Build history of the part. All positions in model axes, mm. Face numbers are marked on the shaded views. A direction names the side the tool comes from. Round coordinates to 2 decimals unless told otherwise and drop trailing zeros. Order: outer loops, then holes, each group sorted by start corner. A loop starts at its lowest first (then second) coordinate and runs counter-clockwise, first axis right, second up. Notation, with made-up numbers: (51.5, -14) - (64.5, -14) arc R14 cw to (64.5, -2) - close; hole circle Ø4 at (-4, -19). An arc over 180 degrees is marked (long way). One line per question, with ' | ' between items. Start each with the question number.
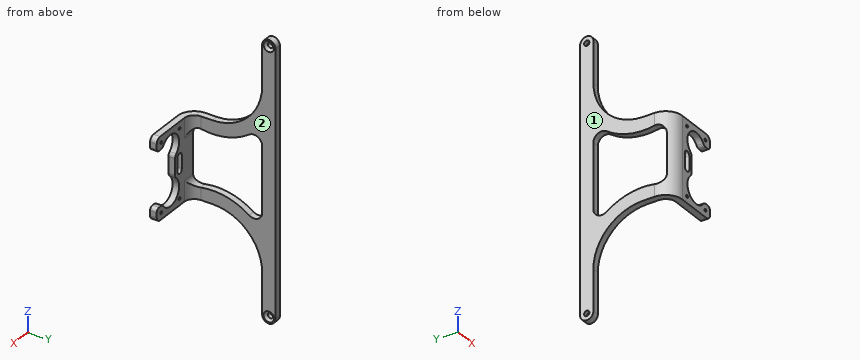
from build123d import *

# Parameters (mm, degrees)
BOSS_EXTRU_1_DEPTH                             = 166
FRAISAGE_POUR_VIS_T_TE_FRAIS_E_M31_D           = 3.2
FRAISAGE_POUR_VIS_T_TE_FRAIS_E_M31_DEPTH       = 4
FRAISAGE_POUR_VIS_T_TE_FRAIS_E_M31_CSINK_D     = 6.3
FRAISAGE_POUR_VIS_T_TE_FRAIS_E_M31_CSINK_ANGLE = 90
D_GAGEMENT_M1_61_D                             = 1.7
D_GAGEMENT_M1_61_DEPTH                         = 4
ENL_V_MAT_EXTRU_1_DEPTH                        = 4
ENL_V_MAT_EXTRU_2_DEPTH                        = 31.75
ENL_V_MAT_EXTRU_2_DEPTH_BACK                   = 5


with BuildPart() as part:
    # Esquisse1 → Boss.-Extru.1 (new body)
    with BuildSketch(Plane.XY):
        with BuildLine():
            Line((0, 0), (-25, 0))
            ThreePointArc((-25, 0), (-32.071067812, 2.928932188), (-35, 10))
            Line((-35, 10), (-35, 55))
            Line((-35, 55), (-31, 55))
            Line((-31, 55), (-31, 10))
            ThreePointArc((-31, 10), (-29.242640687, 5.757359313), (-25, 4))
            Line((-25, 4), (0, 4))
            Line((0, 4), (0, 0))
        make_face()
    extrude(amount=BOSS_EXTRU_1_DEPTH)

    # Fraisage pour vis à tête fraisée M31
    with Locations(Plane(origin=(-31, 0, 0), x_dir=(0, 0, 1), z_dir=(1, 0, 0))):
        with Locations((4, -51), (162, -51)):
            CounterSinkHole(FRAISAGE_POUR_VIS_T_TE_FRAIS_E_M31_D / 2, FRAISAGE_POUR_VIS_T_TE_FRAIS_E_M31_CSINK_D / 2, depth=FRAISAGE_POUR_VIS_T_TE_FRAIS_E_M31_DEPTH, counter_sink_angle=FRAISAGE_POUR_VIS_T_TE_FRAIS_E_M31_CSINK_ANGLE)

    # Dégagement M1.61
    with Locations(Plane(origin=(0, 0, 0), x_dir=(-1, 0, 0), z_dir=(0, -1, 0))):
        with Locations((20.75, -62.5), (20.75, -103.5), (4.25, -103.5), (4.25, -62.5)):
            Hole(D_GAGEMENT_M1_61_D / 2, depth=D_GAGEMENT_M1_61_DEPTH)

    # Esquisse6 → Enlèv. mat.-Extru.1 (cut)
    with BuildSketch(Plane.XZ):
        with BuildLine():
            Line((-35, 58.5), (-3.25, 58.5))
            ThreePointArc((-3.25, 58.5), (-1.128679656, 59.378679656), (-0.25, 61.5))
            Line((-0.25, 61.5), (-0.25, 64.5))
            ThreePointArc((-0.25, 64.5), (-0.835786438, 65.914213562), (-2.25, 66.5))
            Line((-2.25, 66.5), (-3.750142858, 66.5))
            ThreePointArc((-3.750142858, 66.5), (-5.097923909, 66.180202649), (-6.15836042, 65.288990826))
            ThreePointArc((-6.15836042, 65.288990826), (-17.832822404, 64.171534919), (-17.754587156, 75.899094322))
            ThreePointArc((-17.754587156, 75.899094322), (-17.012643745, 76.911706018), (-16.75, 78.139256723))
            Line((-16.75, 78.139256723), (-16.75, 87.860743277))
            ThreePointArc((-16.75, 87.860743277), (-17.012643745, 89.088293982), (-17.754587156, 90.100905678))
            ThreePointArc((-17.754587156, 90.100905678), (-17.832822404, 101.828465081), (-6.15836042, 100.711009174))
            ThreePointArc((-6.15836042, 100.711009174), (-5.097923909, 99.819797351), (-3.750142858, 99.5))
            Line((-3.750142858, 99.5), (-2.25, 99.5))
            ThreePointArc((-2.25, 99.5), (-0.835786438, 100.085786438), (-0.25, 101.5))
            Line((-0.25, 101.5), (-0.25, 104.5))
            ThreePointArc((-0.25, 104.5), (-1.128679656, 106.621320344), (-3.25, 107.5))
            Line((-3.25, 107.5), (-35, 107.5))
            Line((-35, 107.5), (-35, 166))
            Line((-35, 166), (0, 166))
            Line((0, 166), (0, 0))
            Line((0, 0), (-35, 0))
            Line((-35, 0), (-35, 58.5))
        make_face()
        with BuildLine():
            Line((-18.75, 87), (-18.75, 79))
            ThreePointArc((-18.75, 79), (-20.75, 77), (-22.75, 79))
            Line((-22.75, 79), (-22.75, 87))
            ThreePointArc((-22.75, 87), (-20.75, 89), (-18.75, 87))
        make_face()
    extrude(amount=-ENL_V_MAT_EXTRU_1_DEPTH, mode=Mode.SUBTRACT)

    # Esquisse7 → Enlèv. mat.-Extru.2 (cut, two sides)
    with BuildSketch(Plane(origin=(-31, 0, 0), x_dir=(0, 0, -1), z_dir=(1, 0, 0))) as enl_v_mat_extru_2_sk:
        with BuildLine():
            ThreePointArc((-4, 55), (-1.171572875, 53.828427125), (0, 51))
            Line((0, 51), (0, 55))
            Line((0, 55), (-4, 55))
        make_face()
        with BuildLine():
            Line((0, 4), (0, 51))
            ThreePointArc((0, 51), (-1.171572875, 48.171572875), (-4, 47))
            Line((-4, 47), (-28.5, 47))
            ThreePointArc((-28.5, 47), (-49.713203436, 38.213203436), (-58.5, 17))
            Line((-58.5, 17), (-58.5, 4))
            Line((-58.5, 4), (0, 4))
        make_face()
        with BuildLine():
            ThreePointArc((-162, 47), (-164.828427125, 48.171572875), (-166, 51))
            Line((-166, 51), (-166, 4))
            Line((-166, 4), (-107.5, 4))
            Line((-107.5, 4), (-107.5, 17))
            ThreePointArc((-107.5, 17), (-116.286796564, 38.213203436), (-137.5, 47))
            Line((-137.5, 47), (-162, 47))
        make_face()
        with BuildLine():
            Line((-166, 55), (-166, 51))
            ThreePointArc((-166, 51), (-164.828427125, 53.828427125), (-162, 55))
            Line((-162, 55), (-166, 55))
        make_face()
        with BuildLine():
            Line((-63.485711369, 47), (-102.514288631, 47))
            ThreePointArc((-102.514288631, 47), (-106.960347769, 44.287478555), (-106.582394604, 39.093023256))
            ThreePointArc((-106.582394604, 39.093023256), (-100.388347981, 25.168554611), (-100.163444343, 9.930232558))
            ThreePointArc((-100.163444343, 9.930232558), (-99.101139812, 5.810263552), (-95.250739651, 4))
            Line((-95.250739651, 4), (-70.749260349, 4))
            ThreePointArc((-70.749260349, 4), (-66.898860188, 5.810263552), (-65.836555657, 9.930232558))
            ThreePointArc((-65.836555657, 9.930232558), (-65.611652019, 25.168554611), (-59.417605396, 39.093023256))
            ThreePointArc((-59.417605396, 39.093023256), (-59.039652231, 44.287478555), (-63.485711369, 47))
        make_face()
    extrude(amount=ENL_V_MAT_EXTRU_2_DEPTH, mode=Mode.SUBTRACT)
    extrude(enl_v_mat_extru_2_sk.sketch, amount=-ENL_V_MAT_EXTRU_2_DEPTH_BACK, mode=Mode.SUBTRACT)


solid = part.part
Item 1: Slice it at B-B (y = 14). Write the cut outline in (x, z).
Item 2: Slice it at C-C (z = 24.5). Write the cut outline in (x, y).
Item 3: Slice it at A-A (x = -12.5). Write the cut outline in (y, z).
Item 4: Pin check, flat tips, straight feed: pin 1 (20.5 mm diameter, centred on x = -12.5, z = 70, fed in from +Y); pin 2 (13.5 mm diameter, centred on x = -22, y = 8.5, fed in from +Z); pin 3 (6 mm diameter, centred on x = -9.5, z = 69.5, fed in from -Y); pin 4 (1.2 mm diameter, centred on y = 2, z = 85, fed in from +X). Stop position of each tip, or through.
Item 5: 3-axis set-ups, long thin cutter, end or side, ignore diameter. For the marked faces 1 and 2: which of +Z, -Z, +X, -X, +Y, -Y reach the whole face in a straight line?
Item 6: Wall check: line 1 along Z through (x, y) = (-33, 51); line 2 along Z through (x, y) = (-20.75, 1.6); line 3 along Z through (x, y) = (-4.25, 1.8). Give the ranges that are in metal, low to high. Write a range as [from, to].
A:
1) outline: (-35, 58.5) - (-31, 58.5) - (-31, 66.38) - (-35, 66.38) - close; (-35, 99.62) - (-31, 99.62) - (-31, 107.5) - (-35, 107.5) - close
2) outline: (-35, 47) - (-31, 47) - (-31, 55) - (-35, 55) - close
3) outline: (0, 58.5) - (4, 58.5) - (4, 62.1) - (0, 62.1) - close; (0, 103.9) - (4, 103.9) - (4, 107.5) - (0, 107.5) - close
4) pin 1: y = 4 | pin 2: z = 107.5 | pin 3: through | pin 4: x = -16.75
5) face 1: +Z, -Z, -X, +Y, -Y | face 2: +Z, -Z, +X, +Y
6) line 1: [0, 2.4], [5.6, 160.4], [163.6, 166] | line 2: [58.5, 61.65], [63.35, 77], [89, 102.65], [104.35, 107.5] | line 3: [58.5, 61.65], [63.35, 66.46], [99.54, 102.65], [104.35, 107.5]
